Print and shaded views of the part. All mm, measured from the part's lowest x, y and z. Coordinates: 2 decimals unless noted, no trailing zeros. Write each loop counter-clockwise with the first axis right and the second up, starting at its lowest first coordinate (ties: lowest second). Pieces come first, ordered by that corner, then holes. Notation, with made-up numbers: (17, 17.5) -> (65, 17.5) arc R8 ccw to (65, 27.5) -> close; hole circle Ø10 at (23, -29). An arc over 180 degrees is marked (long way). Write item = value, one per line.
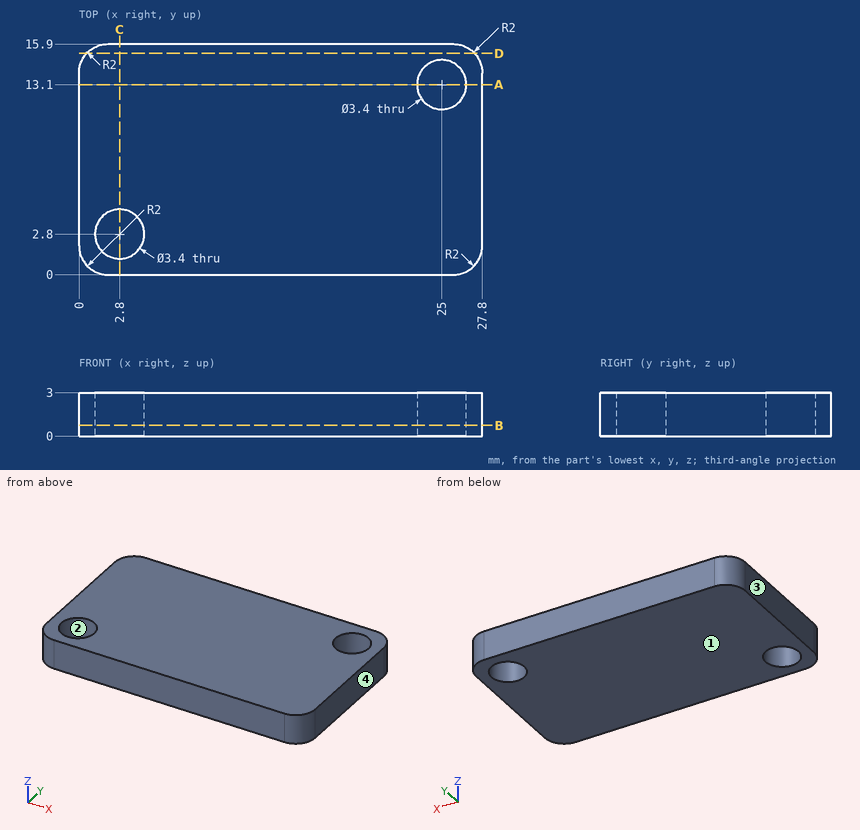
Q1. Probe line 1 (Y direction, x = 25, z = 1.75); line 2 (X direction, y = 13, z = 0.4); line 3 (X direction, y = 3, z = 0.4). List the from-to ranges inside material, lowest first. Write a range as from..to.
Model answer:
line_1 = 0..11.4, 14.8..15.9
line_2 = 0..23.3, 26.7..27.8
line_3 = 0..1.11, 4.49..27.8
Q2. Saw through at D-D on y = 15.25. Give the cut face in (x, z), and give its area (3 significant figures).
Model answer:
outline = (0.52, 0) -> (27.28, 0) -> (27.28, 3) -> (0.52, 3) -> close
area = 80.3 mm²
Q3. Mould opens along X. For the marked faces 1, 2, 3 and 4 say: released by +X, released by -X, zero draft, split by the parting line, or undercut.
Model answer:
face_1 = zero draft
face_2 = undercut
face_3 = released by -X
face_4 = released by +X
Q4. Saw through at C-C on x = 2.8. Give the cut face in (y, z).
Model answer:
outline = (0, 0) -> (1.1, 0) -> (1.1, 3) -> (0, 3) -> close; (4.5, 0) -> (15.9, 0) -> (15.9, 3) -> (4.5, 3) -> close
Q5. Saw through at A-A on y = 13.1. Give the cut face in (x, z), and give its area (3 significant figures).
Model answer:
outline = (0, 0) -> (23.3, 0) -> (23.3, 3) -> (0, 3) -> close; (26.7, 0) -> (27.8, 0) -> (27.8, 3) -> (26.7, 3) -> close
area = 73.2 mm²
Q6. Pin check, flat tip, straight feed: pin 1 (3 mm diameter, centred on x = 2.8, y = 2.8, fed in from -Z). Stop position of the tip, or through.
Model answer:
pin_1 = through
Q7. Saw through at B-B on z = 0.75. Give the cut face in (x, y).
Model answer:
outline = (0, 2) arc R2 ccw to (2, 0) -> (25.8, 0) arc R2 ccw to (27.8, 2) -> (27.8, 13.9) arc R2 ccw to (25.8, 15.9) -> (2, 15.9) arc R2 ccw to (0, 13.9) -> close; hole circle Ø3.4 at (2.8, 2.8); hole circle Ø3.4 at (25, 13.1)
